Input: part model. Units: mm. Frame: model coordinates. Face numbers are marked on the shaded views. A direction names the side the tool comes from. Round coordinates to 2 decimals unless told otherwise and drop trailing zeros. Write each loop counter-clockwise with the first axis right and the second up, starting at its lowest first coordinate (ties: lowest second). Pieces come first, ordered by that corner, then holes. Notation, with made-up numbers: (69.5, -39) -> (95.5, -39) arc R25 ccw to (95.5, -16) -> close; hole circle Ø7 at (43.25, 63). An arc over 180 degrees is marked (long way). Write item = value, one per line. Start each with the question number.
```python
from build123d import *

# Parameters (mm, degrees)
F0_R     = 2.125
F1_DEPTH = 5
F3_DEPTH = 15
F4_SIZE  = 10
F5_R     = 2.125
F6_DEPTH = 5
F7_R     = 2.125
F8_DEPTH = 5
F9_R     = 5


with BuildPart() as f1:
    # F0 (on Top) → F1 (new body)
    with BuildSketch(Plane.XY):
        Polygon((0, 20), (0, 40), (-20, 40), (-20, 0), (20, 0), (20, 20), align=None)
        with Locations((10, 12.5)):
            Circle(F0_R, mode=Mode.SUBTRACT)
        with Locations((-7.5, 30)):
            Circle(F0_R, mode=Mode.SUBTRACT)
    extrude(amount=F1_DEPTH)

    # F2 (on face) → F3 (join)
    with BuildSketch(Plane.XY.offset(5)):
        Polygon((-15, 40), (-20, 40), (-20, 0), (20, 0), (20, 5), (-15, 5), align=None)
    extrude(amount=F3_DEPTH)

    # F4
    f4_edges = [f1.edges().sort_by_distance(p)[0] for p in [
        (0, 20, 2.5),
    ]]
    chamfer(f4_edges, length=F4_SIZE)

    # F5 (on face) → F6 (cut)
    with BuildSketch(Plane.XZ):
        with Locations((10, 12.5)):
            Circle(F5_R)
    extrude(amount=-F6_DEPTH, mode=Mode.SUBTRACT)

    # F7 (on face) → F8 (cut)
    with BuildSketch(Plane(origin=(-20, 0, 0), x_dir=(0, -1, 0), z_dir=(-1, 0, 0))):
        with Locations((-30, 12.5)):
            Circle(F7_R)
    extrude(amount=-F8_DEPTH, mode=Mode.SUBTRACT)

    # F9
    f9_edges = [f1.edges().sort_by_distance(p)[0] for p in [
        (-20, 0, 10),
    ]]
    fillet(f9_edges, radius=F9_R)


solid = f1.part
```
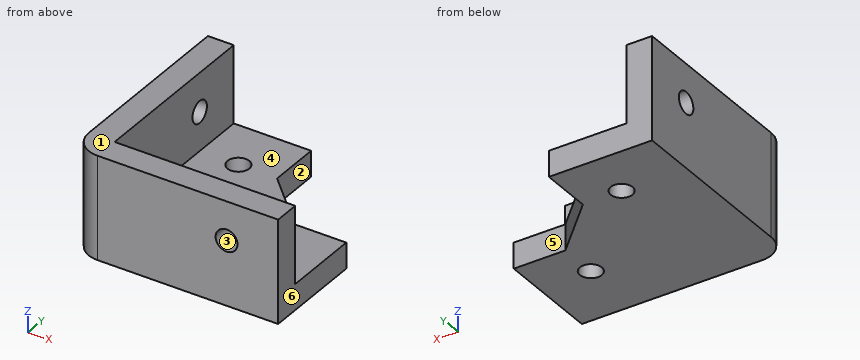
1. Section C-C (z = 3.75). Output: boundary loops of the cut face in (x, y) (3 decimals).
2. Mould query, pull axis X, two halves, no side actions, for the marked faces 1, 2 and 3. Classes: pulls with the +X half, pulls with the -X half, needs draft (parallel to the pull), parting line crosses it, or undercut.
3. Section B-B (y = 12.5). Output: boundary loops of the cut face in (x, z) (3 decimals), then the cut area to 3 significant figures.
4. Pin query (flat end, axial travel): P1, Ø7.5, axis at y = 18.5, z = 14.5, coming from the +X side; P2, Ø5.5, axis at x = 10, z = 12.5, coming from the +Y side; P3, Ø4, axis at x = 13, z = 3, coming from the +Y side. Return the tip coordinate at first contact, or that it passes through.
5. Line query: line 1 along Z through (x, y) = (10, 1.75) (3 decimals); line 2 along Y through (x, z) = (-9.5, 11). Output: solid intervals per line, ascending.
6. Reachability of the marked faces 4, 5 and 6 from +Z, -Z, +X, -X, +Y, -Y: full face, straight path, thin tool, end or side. Return the list, or none.
7. Section D-D (y = 29.5). Output: boundary loops of the cut face in (x, z).
8. Section A-A (z = 12.5). Output: boundary loops of the cut face in (x, y) (3 decimals).
Check sheet entries:
q1.outline = (-20, 5) arc R5 ccw to (-15, 0) -> (20, 0) -> (20, 20) -> (10, 20) -> (0, 30) -> (0, 40) -> (-20, 40) -> close; hole circle Ø4.25 at (-7.5, 30); hole circle Ø4.25 at (10, 12.5)
q2.face_1 = needs draft
q2.face_2 = pulls with the +X half
q2.face_3 = undercut
q3.outline = (-20, 0) -> (7.875, 0) -> (7.875, 5) -> (-15, 5) -> (-15, 20) -> (-20, 20) -> close; (12.125, 0) -> (20, 0) -> (20, 5) -> (12.125, 5) -> close
q3.area = 254 mm2
q4.P1 = -15
q4.P2 = 5
q4.P3 = 20
q5.line_1 = 0 to 10.375, 14.625 to 20
q5.line_2 = 0 to 5
q6.face_4 = +Z, +X, +Y
q6.face_5 = +Z, -Z, +X, +Y
q6.face_6 = +Z, -Z, +X, +Y, -Y
q7.outline = (-20, 0) -> (-9.57, 0) -> (-9.57, 5) -> (-15, 5) -> (-15, 10.43) -> (-20, 10.43) -> close; (-20, 14.57) -> (-15, 14.57) -> (-15, 20) -> (-20, 20) -> close; (-5.43, 0) -> (0.5, 0) -> (0.5, 5) -> (-5.43, 5) -> close
q8.outline = (-20, 5) arc R5 ccw to (-15, 0) -> (7.875, 0) -> (7.875, 5) -> (-15, 5) -> (-15, 27.875) -> (-20, 27.875) -> close; (-20, 32.125) -> (-15, 32.125) -> (-15, 40) -> (-20, 40) -> close; (12.125, 0) -> (20, 0) -> (20, 5) -> (12.125, 5) -> close
